Work out the finished part from the listing and answer in its coordinate system (mm). Face numbers are marked on the shaded views. A direction names the side the tool comes from. Round coordinates to 2 decimals unless told otherwise and drop trailing zeros. Loops run counter-clockwise (first coordinate to the right, second up) from the corner with the lowest first, then second, coordinate; pieces in that order, holes last.
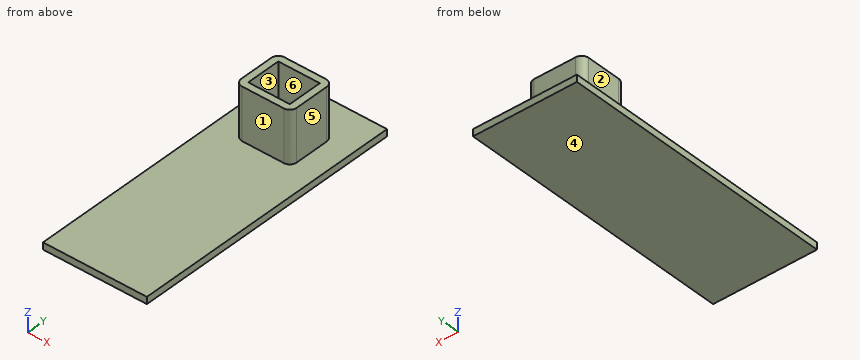
```python
from build123d import *

# Parameters (mm, degrees)
SKETCH_1_W      = 30
SKETCH_1_H      = 80
EXTRUDE_1_DEPTH = 2
SKETCH_2_W      = 16
SKETCH_2_H      = 14
SKETCH_2_W_2    = 12
SKETCH_2_H_2    = 10
EXTRUDE_2_DEPTH = 15
FILLET_1_R      = 2


with BuildPart() as part:
    # 草图1 → 凸台-拉伸1 (new body)
    with BuildSketch(Plane.XY):
        with Locations((15, -40)):
            Rectangle(SKETCH_1_W, SKETCH_1_H)
    extrude(amount=EXTRUDE_1_DEPTH)

    # 草图2 → 凸台-拉伸2 (add)
    with BuildSketch(Plane.XY.offset(2)):
        with Locations((15, -17)):
            Rectangle(SKETCH_2_W, SKETCH_2_H)
        with Locations((15, -17)):
            Rectangle(SKETCH_2_W_2, SKETCH_2_H_2, mode=Mode.SUBTRACT)
    extrude(amount=EXTRUDE_2_DEPTH)

    # 圆角1
    fillet_1_edges = [part.edges().sort_by_distance(p)[0] for p in [
        (23, -10, 9.5),
        (7, -10, 9.5),
        (7, -24, 9.5),
        (23, -24, 9.5),
    ]]
    fillet(fillet_1_edges, radius=FILLET_1_R)


solid = part.part
```
1. Given pin 1 (8 mm diameter, centred on y = -16, z = 12, fed in from -X); pin 2 (3.5 mm diameter, centred on x = 13, z = 13, fed in from +Y); pin 3 (8 mm diameter, centred on y = -46.5, z = 8, fed in from -X); pin 4 (3 mm diameter, centred on x = 13, y = -69, fed in from +Z), each flat-ended and moving along its own axis, determine where each tip first touches the part or whether it passes through.
Answer key:
pin 1: stops at x = 7
pin 2: stops at y = -10
pin 3: passes through
pin 4: stops at z = 2
2. Find section B-B (x = 18.5). Write down the section's boundary in (y, z).
Answer key:
outline: (-80, 0) - (0, 0) - (0, 2) - (-10, 2) - (-10, 17) - (-12, 17) - (-12, 2) - (-22, 2) - (-22, 17) - (-24, 17) - (-24, 2) - (-80, 2) - close
3. Determine the mould class of the marked faces 1, 2 and 3 for opening direction Y: +Y half, -Y half, draft (parallel to the pull), parting line (faces both ways), or undercut.
Answer key:
face 1: -Y half
face 2: draft
face 3: undercut
4. Consider probe 1 along X at (y, z) = (-13, 4); probe 2 along Y at (x, z) = (20.5, 5); probe 3 along Z at (x, y) = (12.75, -20). Determine where each line is inside the solid, lowest interval first.
Answer key:
probe 1: x = 7 to 9, 21 to 23
probe 2: y = -24 to -22, -12 to -10
probe 3: z = 0 to 2
5. Which of the six approach directions +Z, -Z, +X, -X, +Y, -Y give full straight-line access (tool end or side, diameter ignored) to the marked faces 4, 5 and 6?
Answer key:
face 4: -Z, +X, -X, +Y, -Y
face 5: +Z, +X, +Y, -Y
face 6: +Z
6. Find section C-C (y = -52). Write down the section's boundary in (x, z).
Answer key:
outline: (0, 0) - (30, 0) - (30, 2) - (0, 2) - close
7. Find section D-D (x = 8). Write down the section's boundary in (y, z), then the cut area to 3 significant figures.
Answer key:
outline: (-80, 0) - (0, 0) - (0, 2) - (-10.27, 2) - (-10.27, 17) - (-23.73, 17) - (-23.73, 2) - (-80, 2) - close
area: 362 mm2
8. Find section A-A (z = 7). Write down the section's boundary in (x, y), then the cut area to 3 significant figures.
Answer key:
outline: (7, -22) arc R2 ccw to (9, -24) - (21, -24) arc R2 ccw to (23, -22) - (23, -12) arc R2 ccw to (21, -10) - (9, -10) arc R2 ccw to (7, -12) - close; hole (9, -22) - (21, -22) - (21, -12) - (9, -12) - close
area: 101 mm2
